Here's the drawing with two shaded views (mm, measured from the low corner). I have some questions. Round coordinates to 2 decimals unless told otherwise and drop trailing zeros. Loops run counter-clockwise (first coordinate to the right, second up) from the corner with the lowest first, then second, coordinate; pieces in that order, holes last.
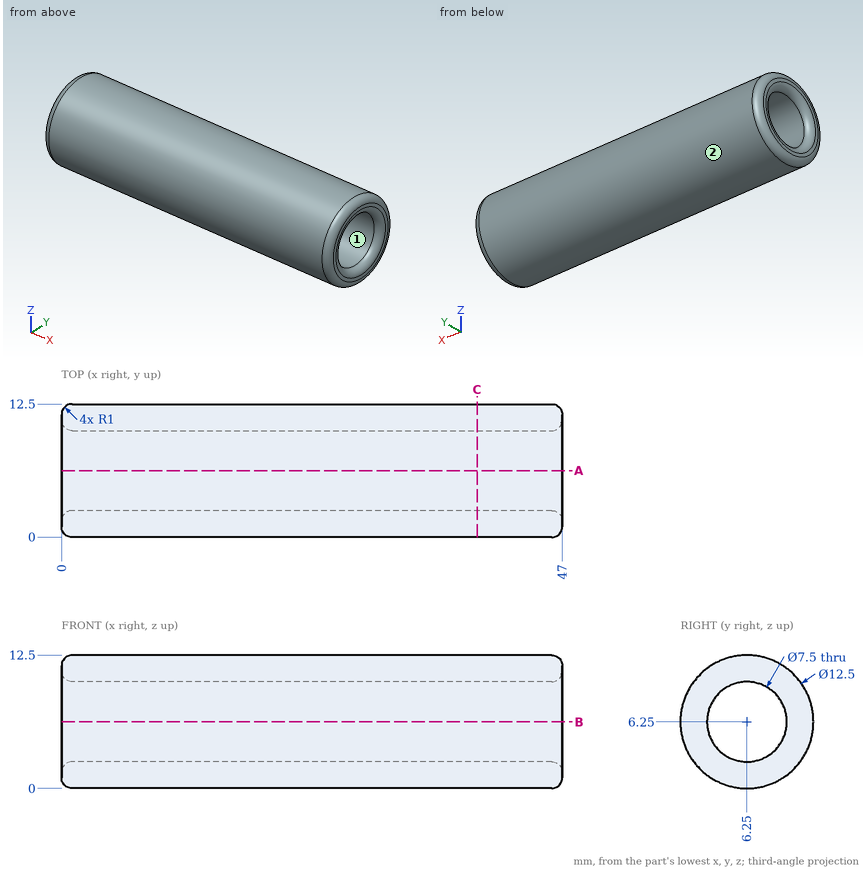
Item 1: Will these pins go through, and if not, where does the flat tip stop? pin 1 (1.5 mm diameter, centred on x = 17.5, z = 9.5, fed in from +Y); pin 2 (1.5 mm diameter, centred on x = 9, z = 9, fed in from -Y); pin 3 (4 mm diameter, centred on x = 14.5, z = 3, fed in from +Y).
Results list:
pin 1: stops at y = 11.98
pin 2: stops at y = 0.33
pin 3: stops at y = 12.37
Item 2: If I drill on line 1 along Z through (x, y) = (36, 6.25); line 2 along Z through (x, y) = (7.5, 5.5); line 3 along Z through (x, y) = (8, 11.25), over which ranges is the centre line in solid material (lowest first)?
Results list:
line 1: z = 0 to 2.5, 10 to 12.5
line 2: z = 0.05 to 2.58, 9.92 to 12.45
line 3: z = 2.5 to 10
Item 3: We'd pull the mould along Z, two halves only. Please class the marked faces 1 and 2: released by +Z, released by -Z, zero draft, split by the parting line, or undercut.
Results list:
face 1: undercut
face 2: split by the parting line
Item 4: If we section it at C-C, the plane x = 39: Please give me the cut outline in (y, z).
Results list:
outline: circle Ø12.5 at (6.25, 6.25); hole circle Ø7.5 at (6.25, 6.25)
Item 5: If we section it at A-A, the plane y = 6.25: Please give me the cut outline in (x, z).
Results list:
outline: (0, 1) arc R1 ccw to (1, 0) - (46, 0) arc R1 ccw to (47, 1) - (47, 1.5) arc R1 ccw to (46, 2.5) - (1, 2.5) arc R1 ccw to (0, 1.5) - close; (0, 11) arc R1 ccw to (1, 10) - (46, 10) arc R1 ccw to (47, 11) - (47, 11.5) arc R1 ccw to (46, 12.5) - (1, 12.5) arc R1 ccw to (0, 11.5) - close
